Could you check a few things on this model? Use its own coordinates, in mm. A direction names the side the tool comes from. Coordinates: 2 decimals unless noted, no trailing zeros. Order: outer loops, then holes, each group sorted by start corner. A loop starts at its lowest first (then second) coordinate and runs counter-clockwise, first axis right, second up. Notation, with made-up numbers: (14, 78.25) -> (28, 78.25) arc R11 cw to (28, 95.25) -> close; hole circle Ø2 at (-21.75, 54.25). An arc over 180 degrees is marked (long way). Return JSON: item names as keys, results as strings. Group by question number.
from build123d import *

# Parameters (mm, degrees)
BOSS_EXTRUDE1_DEPTH = 50
SKETCH3_R           = 5
CUT_EXTRUDE1_DEPTH  = 64
CUT_EXTRUDE2_DEPTH  = 9
SKETCH7_R           = 5
CUT_EXTRUDE3_DEPTH  = 82
SKETCH8_W           = 40
SKETCH8_H           = 12
CUT_EXTRUDE4_DEPTH  = 82
SKETCH9_W           = 10
SKETCH9_H           = 12
CUT_EXTRUDE5_DEPTH  = 82
CUT_EXTRUDE6_DEPTH  = 82
SKETCH11_R          = 25
CUT_EXTRUDE7_DEPTH  = 13
BOSS_EXTRUDE2_DEPTH = 8
BOSS_EXTRUDE3_DEPTH = 5
SKETCH14_R          = 5
BOSS_EXTRUDE4_DEPTH = 8


with BuildPart() as part:
    # Sketch1 → Boss-Extrude1 (new body)
    with BuildSketch(Plane.XY):
        with BuildLine():
            Line((0, 5), (0, 0))
            Line((0, 0), (45, 0))
            Line((45, 0), (71.869067897, 9.497224024))
            ThreePointArc((71.869067897, 9.497224024), (77.313595869, 9.728683064), (82.071067812, 7.071067812))
            Line((82.071067812, 7.071067812), (89.142135624, 0))
            Line((89.142135624, 0), (100, 0))
            Line((100, 0), (100, 48))
            Line((100, 48), (60, 48))
            Line((60, 48), (60, 63))
            Line((60, 63), (30, 63))
            Line((30, 63), (30, 35))
            ThreePointArc((30, 35), (21.213203436, 13.786796564), (0, 5))
        make_face()
    extrude(amount=BOSS_EXTRUDE1_DEPTH)

    # Sketch3 → Cut-Extrude1 (cut)
    with BuildSketch(Plane.XY.offset(50)):
        with Locations((90, 35)):
            Circle(SKETCH3_R)
    extrude(amount=-CUT_EXTRUDE1_DEPTH, mode=Mode.SUBTRACT)

    # Sketch6 → Cut-Extrude2 (cut)
    with BuildSketch(Plane.XY.offset(50)):
        with BuildLine():
            Line((80, 48), (100, 48))
            Line((100, 48), (100, 35))
            Line((100, 35), (100, 15))
            ThreePointArc((100, 15), (85.857864376, 20.857864376), (80, 35))
            Line((80, 35), (80, 48))
        make_face()
    extrude(amount=-CUT_EXTRUDE2_DEPTH, mode=Mode.SUBTRACT)

    # Sketch7 → Cut-Extrude3 (cut)
    with BuildSketch(Plane(origin=(0, 63, 0), x_dir=(1, 0, 0), z_dir=(0, 1, 0))):
        with Locations(Location((39, -20, 0), (0, 0, 180))):
            Circle(SKETCH7_R)
    extrude(amount=-CUT_EXTRUDE3_DEPTH, mode=Mode.SUBTRACT)

    # Sketch8 → Cut-Extrude4 (cut)
    with BuildSketch(Plane(origin=(0, 48, 0), x_dir=(1, 0, 0), z_dir=(0, 1, 0))):
        with Locations((80, -6)):
            Rectangle(SKETCH8_W, SKETCH8_H)
    extrude(amount=-CUT_EXTRUDE4_DEPTH, mode=Mode.SUBTRACT)

    # Sketch9 → Cut-Extrude5 (cut)
    with BuildSketch(Plane(origin=(0, 63, 0), x_dir=(1, 0, 0), z_dir=(0, 1, 0))):
        with Locations((55, -6)):
            Rectangle(SKETCH9_W, SKETCH9_H)
    extrude(amount=-CUT_EXTRUDE5_DEPTH, mode=Mode.SUBTRACT)

    # Sketch10 → Cut-Extrude6 (cut)
    with BuildSketch(Plane(origin=(50, 0, 0), x_dir=(0, 0, -1), z_dir=(1, 0, 0))):
        Polygon((0, 63), (0, 45), (-6.551464217, 63), align=None)
    extrude(amount=-CUT_EXTRUDE6_DEPTH, mode=Mode.SUBTRACT)

    # Sketch11 → Cut-Extrude7 (cut)
    with BuildSketch(Plane.XY.offset(50)):
        with Locations((30, 35)):
            Circle(SKETCH11_R)
    extrude(amount=-CUT_EXTRUDE7_DEPTH, mode=Mode.SUBTRACT)

    # Sketch12 → Boss-Extrude2 (add)
    with BuildSketch(Plane.XY.offset(50)):
        with BuildLine():
            ThreePointArc((19.583333333, 12.273516428), (17.218757327, 13.514194553), (15, 15))
            ThreePointArc((15, 15), (7.90569415, 11.282917549), (0, 10))
            Line((0, 10), (0, 5))
            ThreePointArc((0, 5), (10.445226011, 6.877104459), (19.583333333, 12.273516428))
        make_face()
    extrude(amount=-BOSS_EXTRUDE2_DEPTH)

    # Sketch13 → Boss-Extrude3 (add)
    with BuildSketch(Plane.XY.offset(37)):
        with BuildLine():
            ThreePointArc((28.333333333, 25.139867028), (39.964971895, 34.163737397), (30, 45))
            Line((30, 45), (30, 35))
            ThreePointArc((30, 35), (29.580398915, 30), (28.333333333, 25.139867028))
        make_face()
    extrude(amount=BOSS_EXTRUDE3_DEPTH)

    # Sketch14 → Boss-Extrude4 (add)
    with BuildSketch(Plane.XY.offset(42)):
        with Locations(Location((30, 35, 0), (0, 0, 265.219808153))):
            Circle(SKETCH14_R)
    extrude(amount=BOSS_EXTRUDE4_DEPTH)


solid = part.part
Q1. I want a section at B-B on y = 36.5. Please give me the cut outline in (x, z), and give its area (3 significant figures).
Q2. I want a section at C-C on z = 34. Please give me the cut outline in (x, y), and give its area (3 significant figures).
Q3. We'd pull the mould along X, two halves only. Please class faces 4 (the cylindrical face through (77.238, 9.746, 30.734)), 5 (the flat face through (50, 33, 6)), 6 (the cylindrical face through (94.77, 36.5, 26.7)), 7 (the flat face through (0, 3, 31)): pulls with the +X half, pulls with the -X half, needs draft (parallel to the pull), parting line crosses it, or undercut.
Q4. I want a section at A-A on z = 23. Please give me the cut outline in (x, y), and give its area (3 significant figures).
Q5. I need wall thicknesses on line 1 along Z through (x, y) = (39, 24); line 2 along X through (y, z) = (35, 45); line 3 along Y through (x, z) = (31.5, 38.5). Which ranges of each line are inside material? Lowest first, please. Write a range as from..to.
Q6. On a 3-axis mill with a long thin cutter (end or side, diameter ignored), from which of +Z, -Z, +X, -X, +Y, -Y can I reach the whole of each face in a straight line? I mean faces 1 (the flat face through (41, 30, 37)), 2 (the flat face through (60, 55, 31)), 3 (the flat face through (30, 49, 25)). Say none if no direction works.
Q7. I want a section at D-D on x = 37.5. Please give me the cut outline in (y, z), and give its area (3 significant figures).
Q8. I'm going to push flat-ended pins straight in: pin 1 Ø13 at (y, z) = (27, 5) entering from +X; pin 2 Ø12 at (y, z) = (33.5, 24) entering from -X; pin 3 Ø1.5 at (x, y) = (55.5, 6.5) entering from -Z. Where does each tip first touch, or does it pass through?
Response values:
{
 "1": {"outline": "(25.23, 42) -> (30, 42) -> (30, 0) -> (50, 0) -> (50, 12) -> (85.23, 12) -> (85.23, 41) -> (80, 41) -> (80, 50) -> (54.95, 50) -> (54.95, 37) -> (39.89, 37) -> (39.89, 42) -> (34.77, 42) -> (34.77, 50) -> (25.23, 50) -> close; (94.77, 12) -> (100, 12) -> (100, 41) -> (94.77, 41) -> close; hole circle Ø10 at (39, 20)", "area": "2,170 mm²"},
 "2": {"outline": "(0, 0) -> (45, 0) -> (71.87, 9.5) arc R10 cw to (82.07, 7.07) -> (89.14, 0) -> (100, 0) -> (100, 48) -> (60, 48) -> (60, 63) -> (30, 63) -> (30, 35) arc R30 cw to (0, 5) -> close; hole circle Ø10 at (90, 35)", "area": "3,830 mm²"},
 "3": {"face 4": "undercut", "face 5": "pulls with the +X half", "face 6": "undercut", "face 7": "pulls with the -X half"},
 "4": {"outline": "(0, 0) -> (35, 0) -> (35, 63) -> (30, 63) -> (30, 35) arc R30 cw to (0, 5) -> close; (43, 0) -> (45, 0) -> (71.87, 9.5) arc R10 cw to (82.07, 7.07) -> (89.14, 0) -> (100, 0) -> (100, 48) -> (60, 48) -> (60, 63) -> (43, 63) -> close; hole circle Ø10 at (90, 35)", "area": "3,320 mm²"},
 "5": {"line 1": "z = 0..15, 25..37", "line 2": "x = 25..35, 55..80", "line 3": "y = 0..10.05, 25.11..44.89, 59.95..63"},
 "6": {"face 1": "+Z", "face 2": "+Z, -Z, +X, +Y", "face 3": "-Z, -X, +Y"},
 "7": {"outline": "(0, 0) -> (45, 0) -> (63, 6.55) -> (63, 15.23) -> (0, 15.23) -> close; (0, 24.77) -> (63, 24.77) -> (63, 50) -> (58.85, 50) -> (58.85, 37) -> (41.61, 37) -> (41.61, 42) -> (28.39, 42) -> (28.39, 37) -> (11.15, 37) -> (11.15, 50) -> (0, 50) -> close", "area": "1,940 mm²"},
 "8": {"pin 1": "stops at x = 50", "pin 2": "stops at x = 29.05", "pin 3": "stops at z = 12"}
}
